```python
from build123d import *

# Parameters (mm, degrees)
SKETCH1_W           = 53.34
SKETCH1_H           = 26
BOSS_EXTRUDE1_DEPTH = 1.5
SKETCH2_R           = 0.5
CUT_EXTRUDE1_DEPTH  = 1.5
LPATTERN1_COUNT     = 20
LPATTERN1_PITCH     = 2.54


with BuildPart() as part:
    # Sketch1 → Boss-Extrude1 (new body)
    with BuildSketch(Plane(origin=(0, 0, 0), x_dir=(1, 0, 0), z_dir=(0, 1, 0))):
        with Locations((26.67, 13)):
            Rectangle(SKETCH1_W, SKETCH1_H)
    extrude(amount=BOSS_EXTRUDE1_DEPTH)

    # Sketch2 → Cut-Extrude1 (cut)
    with BuildSketch(Plane(origin=(0, 1.5, 0), x_dir=(1, 0, 0), z_dir=(0, 1, 0))):
        with Locations((2.54, 1.57)):
            Circle(SKETCH2_R)
        with Locations((2.54, 24.43)):
            Circle(SKETCH2_R)
    cut_extrude1 = extrude(amount=-CUT_EXTRUDE1_DEPTH, mode=Mode.SUBTRACT)

    # LPattern1: Cut-Extrude1 ×20
    with Locations(*[(i * LPATTERN1_PITCH, 0, 0) for i in range(1, LPATTERN1_COUNT)]):
        add(cut_extrude1, mode=Mode.SUBTRACT)


solid = part.part
```
Check sheet for the modelled part. Datum: model origin and axes. Units: mm. Give positions to 0.01 mm unless a question says otherwise; leave off trailing zeros. Write each loop counter-clockwise with the first axis right and the second up, starting at its lowest first coordinate (ties: lowest second). Pieces come first, ordered by that corner, then holes. Notation, with made-up numbers: (22, 65) - (26, 65) arc R29 cw to (26, 101) - close; hole circle Ø1 at (60.25, 64). An arc over 180 degrees is marked (long way). Answer as a JSON object with one key per item and string values. Group by question number.
1) Release check for a two-part mould opening along X. For faces 1 (the face through (40.871, 0.76, -23.986)), 2 (the face through (26, 0, -13)) record: pulls with the +X half, pulls with the -X half, needs draft (parallel to the pull), parting line crosses it, or undercut.
2) Sectioned sample at B-B (z = -24.43). Give the number of separate pieces and of enclosed holes in the cut face, then the cut area to 3 significant figures.
3) Sectioned sample at A-A (x = 45.72). Record the cut outline in (y, z), then the cut area to 3 significant figures.
4) Thickness scan on probe 1 along Z at (x, y) = (43.18, 0.4); probe 2 along Z at (x, y) = (43, 0.1). Record the ranges inside material, lowest first. Write a range as from..to.
Geometry results:
{
 "1": {"face 1": "undercut", "face 2": "needs draft"},
 "2": {"separate pieces": "21", "enclosed holes": "0", "area": "50.0 mm^2"},
 "3": {"outline": "(0, -26) - (1.5, -26) - (1.5, -24.93) - (0, -24.93) - close; (0, -23.93) - (1.5, -23.93) - (1.5, -2.07) - (0, -2.07) - close; (0, -1.07) - (1.5, -1.07) - (1.5, 0) - (0, 0) - close", "area": "36.0 mm^2"},
 "4": {"probe 1": "z = -26..-24.93, -23.93..-2.07, -1.07..0", "probe 2": "z = -26..-24.9, -23.96..-2.04, -1.1..0"}
}
